Read the model definition and answer for the solid it produces. Units are mm, in the model's axes. Give positions to 0.01 mm unless a question says otherwise; leave off trailing zeros. Loops run counter-clockwise (first coordinate to the right, second up) from the corner with the lowest first, then second, coordinate; pieces in that order, holes last.
(1) Find section B-B, the plane x = 26.5. Write down the section's boundary in (y, z).
(2) Find section C-C, the plane z = -57. Write down the section's boundary in (x, y), then the cut area to 3 significant figures.
(3) Each of these flat-tipped pins is pushed along its axis until it touches: P1, Ø12, axis at x = -14, y = -6, coming from the +Z side; P2, Ø10, axis at y = -20.5, z = 29.5, coming from the +X side; P3, Ø2, axis at y = -8, z = -51, coming from the -X side. Where does it stop, or does it pass through?
(4) Straight lines are drawn through the part: probe 1 along Z at (x, y) = (-1, -10.5); probe 2 along X at (y, z) = (-8.75, 36.5); probe 3 along Z at (x, y) = (41, -11.5). For each, find the intervals that lie inside material, in ascending order.
(5) Find section A-A, the plane y = -17.25. Write down the section's boundary in (x, z), then the cut area to 3 significant figures.
```python
from build123d import *

# Parameters (mm, degrees)
F1_DEPTH = 25.4
F0_W     = 2.0122602582
F0_H     = 9.6141556278
F0_W_2   = 9.3905702233
F0_H_2   = 4.6952851117
F0_H_3   = 17.2160472721
F0_W_3   = 2.6830211282
F0_H_4   = 3.1301882118
F0_W_4   = 1.7886832356
F0_H_5   = 10.0613348186


with BuildPart() as f1:
    # F0 (on Front) → F1 (new body)
    with BuildSketch(Plane.XZ):
        with BuildLine():
            ThreePointArc((74.1845954161, 0), (-38.8508509686, 63.1978288873), (-33.4918178247, -66.1940506076))
            ThreePointArc((-33.4918178247, -66.1940506076), (38.8508509686, -63.1978288873), (74.1845954161, 0))
        make_face()
        with BuildLine():
            ThreePointArc((53.2162221936, 0), (27.8696069711, -45.3348796385), (-24.0253115762, -47.4842153586))
            ThreePointArc((-24.0253115762, -47.4842153586), (-27.8696069711, 45.3348796385), (53.2162221936, 0))
        make_face(mode=Mode.SUBTRACT)
        with BuildLine():
            ThreePointArc((53.2162221936, 0), (-27.8696069711, 45.3348796385), (-24.0253115762, -47.4842153586))
            ThreePointArc((-24.0253115762, -47.4842153586), (27.8696069711, -45.3348796385), (53.2162221936, 0))
        make_face()
        with BuildLine():
            ThreePointArc((40.3185295406, 0), (21.1150195491, -34.3473401263), (-18.2024426872, -35.9757543984))
            ThreePointArc((-18.2024426872, -35.9757543984), (-21.1150195491, 34.3473401263), (40.3185295406, 0))
        make_face(mode=Mode.SUBTRACT)
        with BuildLine():
            ThreePointArc((40.3185295406, 0), (-21.1150195491, 34.3473401263), (-18.2024426872, -35.9757543984))
            ThreePointArc((-18.2024426872, -35.9757543984), (21.1150195491, -34.3473401263), (40.3185295406, 0))
        make_face()
        with BuildLine():
            ThreePointArc((30.8835030596, 0), (16.1738480614, -26.3096446216), (-13.9428496234, -27.5569901406))
            ThreePointArc((-13.9428496234, -27.5569901406), (-16.1738480614, 26.3096446216), (30.8835030596, 0))
        make_face(mode=Mode.SUBTRACT)
        with BuildLine():
            ThreePointArc((30.8835030596, 0), (-16.1738480614, 26.3096446216), (-13.9428496234, -27.5569901406))
            ThreePointArc((-13.9428496234, -27.5569901406), (16.1738480614, -26.3096446216), (30.8835030596, 0))
        make_face()
        with BuildLine():
            ThreePointArc((23.2248742524, 0), (12.1629850953, -19.7852616261), (-10.4852395986, -20.723284841))
            ThreePointArc((-10.4852395986, -20.723284841), (-12.1629850953, 19.7852616261), (23.2248742524, 0))
        make_face(mode=Mode.SUBTRACT)
        with BuildLine():
            ThreePointArc((23.2248742524, 0), (-12.1629850953, 19.7852616261), (-10.4852395986, -20.723284841))
            ThreePointArc((-10.4852395986, -20.723284841), (12.1629850953, -19.7852616261), (23.2248742524, 0))
        make_face()
        with BuildLine():
            ThreePointArc((17.4618084215, 0), (9.1448381274, -14.8757080158), (-7.8834116876, -15.5809683111))
            ThreePointArc((-7.8834116876, -15.5809683111), (-9.1448381274, 14.8757080158), (17.4618084215, 0))
        make_face(mode=Mode.SUBTRACT)
        with BuildLine():
            ThreePointArc((17.4618084215, 0), (-9.1448381274, 14.8757080158), (-7.8834116876, -15.5809683111))
            ThreePointArc((-7.8834116876, -15.5809683111), (9.1448381274, -14.8757080158), (17.4618084215, 0))
        make_face()
        with BuildLine():
            ThreePointArc((13.1806981516, 0), (6.902798845, -11.2286317898), (-5.9506362314, -11.760983471))
            ThreePointArc((-5.9506362314, -11.760983471), (-6.902798845, 11.2286317898), (13.1806981516, 0))
        make_face(mode=Mode.SUBTRACT)
        with BuildLine():
            ThreePointArc((13.1806981516, 0), (-6.902798845, 11.2286317898), (-5.9506362314, -11.760983471))
            ThreePointArc((-5.9506362314, -11.760983471), (6.902798845, -11.2286317898), (13.1806981516, 0))
        make_face()
        with BuildLine():
            ThreePointArc((-4.1793532864, -8.2601763927), (-4.8480925259, 7.8862859948), (9.2572948495, 0))
            ThreePointArc((9.2572948495, 0), (4.8480925259, -7.8862859948), (-4.1793532864, -8.2601763927))
        make_face(mode=Mode.SUBTRACT)
        with BuildLine():
            ThreePointArc((-4.1793532864, -8.2601763927), (4.8480925259, -7.8862859948), (9.2572948495, 0))
            ThreePointArc((9.2572948495, 0), (-4.8480925259, 7.8862859948), (-4.1793532864, -8.2601763927))
        make_face()
        with BuildLine():
            ThreePointArc((6.7578094068, 0), (3.5390992519, -5.7569752877), (-3.0509207508, -6.0299146387))
            ThreePointArc((-3.0509207508, -6.0299146387), (-3.5390992519, 5.7569752877), (6.7578094068, 0))
        make_face(mode=Mode.SUBTRACT)
        with BuildLine():
            ThreePointArc((6.7578094068, 0), (-3.5390992519, 5.7569752877), (-3.0509207508, -6.0299146387))
            ThreePointArc((-3.0509207508, -6.0299146387), (3.5390992519, -5.7569752877), (6.7578094068, 0))
        make_face()
        with BuildLine():
            ThreePointArc((5.0579216156, 0), (2.648859346, -4.3088415188), (-2.2834793176, -4.5131245579))
            ThreePointArc((-2.2834793176, -4.5131245579), (-2.648859346, 4.3088415188), (5.0579216156, 0))
        make_face(mode=Mode.SUBTRACT)
        with BuildLine():
            ThreePointArc((5.0579216156, 0), (-2.648859346, 4.3088415188), (-2.2834793176, -4.5131245579))
            ThreePointArc((-2.2834793176, -4.5131245579), (2.648859346, -4.3088415188), (5.0579216156, 0))
        make_face()
        with BuildLine():
            ThreePointArc((2.9671045807, 0), (1.5538878015, -2.5276752745), (-1.3395466475, -2.6475128653))
            ThreePointArc((-1.3395466475, -2.6475128653), (-1.5538878015, 2.5276752745), (2.9671045807, 0))
        make_face(mode=Mode.SUBTRACT)
        with BuildLine():
            ThreePointArc((2.9671045807, 0), (-1.5538878015, 2.5276752745), (-1.3395466475, -2.6475128653))
            ThreePointArc((-1.3395466475, -2.6475128653), (1.5538878015, -2.5276752745), (2.9671045807, 0))
        make_face()
    extrude(amount=F1_DEPTH)


with BuildPart() as f1b:
    # F0 (on Front) → F1, piece 2 (new body)
    with BuildSketch(Plane.XZ):
        Polygon((81.161364913, -32.4920788407), (81.161364913, -71.3958665729), (103.0726954341, -71.3958665729), (103.0726954341, -32.4920788407), (100.3896817565, -32.4920788407), (95.9179773927, -32.4920788407), align=None)
        Polygon((81.161364913, -1.860929653), (81.161364913, -32.4920788407), (95.9179773927, -32.4920788407), (95.9179773927, -11.4750852808), (95.9179773927, -1.860929653), (84.5151394606, -1.860929653), align=None)
        Polygon((84.5151394606, 21.3919151574), (84.5151394606, -1.860929653), (95.9179773927, -1.860929653), (97.9302376509, -1.860929653), (97.9302376509, 16.2494592369), (97.9302376509, 21.3919151574), (87.8689140081, 21.3919151574), align=None)
        Polygon((87.8689140081, 39.5023003221), (87.8689140081, 21.3919151574), (97.9302376509, 21.3919151574), (97.9302376509, 39.5023003221), (95.9179773927, 39.5023003221), (92.8995758295, 39.5023003221), (90.1047661901, 39.5023003221), align=None)
        Polygon((97.9302376509, -11.4750852808), (100.3896817565, -11.4750852808), (100.3896817565, 16.2494592369), (97.9302376509, 16.2494592369), (97.9302376509, -1.860929653), align=None)
        with Locations((96.9241075218, -6.6680074669)):
            Rectangle(F0_W, F0_H)
        Polygon((95.9179773927, -11.4750852808), (95.9179773927, -32.4920788407), (100.3896817565, -32.4920788407), (100.3896817565, -11.4750852808), (97.9302376509, -11.4750852808), align=None)
    extrude(amount=F1_DEPTH)


with BuildPart() as f1c:
    # F0 (on Front) → F1, piece 3 (new body)
    with BuildSketch(Plane.XZ):
        Polygon((-104.4142097235, 19.3796493113), (-104.4142097235, 22.5098375231), (-109.5566675067, 22.5098375231), (-109.5566675067, -30.7033965364), (-87.1981605887, -30.7033965364), (-87.1981605887, 5.7409610599), (-95.0236395001, 5.7409610599), (-95.0236395001, 19.3796493113), align=None)
        with Locations((-99.7189246118, 42.073527351)):
            Rectangle(F0_W_2, F0_H_2)
        Polygon((-87.1981605887, 22.5098375231), (-92.340618372, 22.5098375231), (-92.340618372, 19.3796493113), (-95.0236395001, 19.3796493113), (-95.0236395001, 5.7409610599), (-87.1981605887, 5.7409610599), align=None)
        Polygon((-108.8859140873, 39.7258847952), (-104.4142097235, 39.7258847952), (-104.4142097235, 44.4211699069), (-95.0236395001, 44.4211699069), (-95.0236395001, 54.4825047255), (-108.8859140873, 54.4825047255), align=None)
        Polygon((-93.2349562645, 54.4825047255), (-93.2349562645, 44.4211699069), (-92.340618372, 44.4211699069), (-92.340618372, 22.5098375231), (-87.1981605887, 22.5098375231), (-87.1981605887, 5.7409610599), (-86.5273997188, 5.7409610599), (-86.5273997188, 59.4013724476), (-95.0236395001, 59.4013724476), (-95.0236395001, 54.4825047255), align=None)
        with Locations((-99.7189246118, 31.1178611591)):
            Rectangle(F0_W_2, F0_H_3)
        with Locations((-93.6821289361, 20.9447434172)):
            Rectangle(F0_W_3, F0_H_4)
        with Locations((-99.7189246118, 20.9447434172)):
            Rectangle(F0_W_2, F0_H_4)
        with Locations((-94.1292978823, 42.073527351)):
            Rectangle(F0_W_4, F0_H_2)
        with Locations((-94.1292978823, 49.4518373162)):
            Rectangle(F0_W_4, F0_H_5)
        Polygon((-93.2349562645, 44.4211699069), (-93.2349562645, 39.7258847952), (-95.0236395001, 39.7258847952), (-95.0236395001, 22.5098375231), (-92.340618372, 22.5098375231), (-92.340618372, 44.4211699069), align=None)
    extrude(amount=F1_DEPTH)


solid = f1.part
```
Entries:
1. outline: (-25.4, -69.29) - (0, -69.29) - (0, 69.29) - (-25.4, 69.29) - close
2. outline: (-47.48, -25.4) - (47.48, -25.4) - (47.48, 0) - (-47.48, 0) - close
2. area: 2,410 mm2
3. P1: stops at z = 73.75
3. P2: stops at x = 70.02
3. P3: stops at x = -54.8
4. probe 1: z = -74.18 to 74.18
4. probe 2: x = -64.58 to 64.58
4. probe 3: z = -61.83 to 61.83
5. outline: circle Ø148.37 at (0, 0)
5. area: 17,300 mm2
